Answer from the drawing. Dimensions are ordinates in mm from the lowest x, y and z of the part. Coordinates: 2 decimals unless noted, no trailing zeros. Write each loop counter-clockwise with the first axis right and the second up, starting at its lowest first coordinate (ties: lowest second). Pieces come first, ordered by that corner, then holes.
1) This flat-tipped pin is pushed along its axis until it touches: pin 1 Ø2 at (x, z) = (7.5, 21.5) entering from -Y. Where does it stop, or does it pass through?
2) The part is cut by section C-C (y = 1.25). Determine the outline of the cut face in (x, z), then the cut area to 3 significant figures.
3) The part is cut by section B-B (x = 7.62). Determine the outline of the cut face in (y, z).
4) Find the intervals of material crossed by line 1 (X direction, y = 3.5, z = 12.7); line 2 (Z direction, x = 7.62, y = 2.5); line 3 (X direction, y = 5, z = 9.75), in increasing order.
5) The part is cut by section A-A (z = 12.7). Determine the outline of the cut face in (x, y), then the cut area to 3 significant figures.
6) Determine the mould class of the marked faces 1, 2 and 3 for opening direction X: +X half, -X half, draft (parallel to the pull), parting line (faces both ways), or undercut.
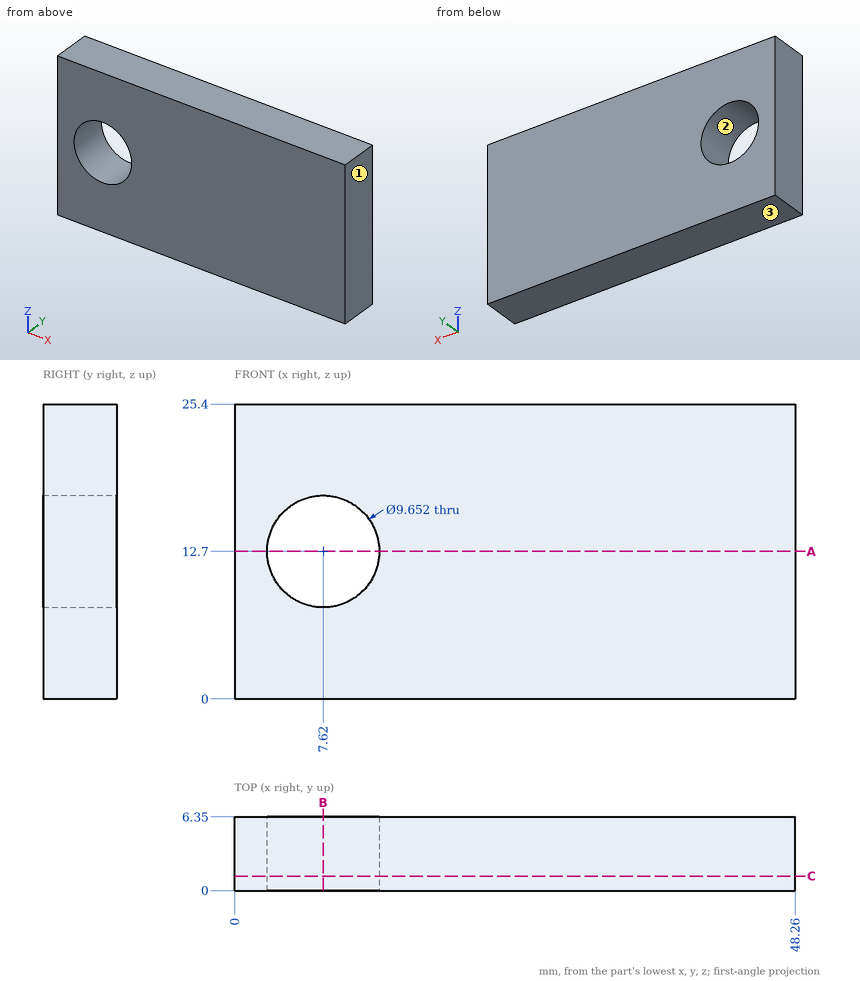
Reported:
1. pin 1: stops at y = 0
2. outline: (0, 0) - (48.26, 0) - (48.26, 25.4) - (0, 25.4) - close; hole circle Ø9.65 at (7.62, 12.7)
2. area: 1,150 mm2
3. outline: (0, 0) - (6.35, 0) - (6.35, 7.87) - (0, 7.87) - close; (0, 17.53) - (6.35, 17.53) - (6.35, 25.4) - (0, 25.4) - close
4. line 1: x = 0 to 2.79, 12.45 to 48.26
4. line 2: z = 0 to 7.87, 17.53 to 25.4
4. line 3: x = 0 to 3.8, 11.44 to 48.26
5. outline: (0, 0) - (2.79, 0) - (2.79, 6.35) - (0, 6.35) - close; (12.45, 0) - (48.26, 0) - (48.26, 6.35) - (12.45, 6.35) - close
5. area: 245 mm2
6. face 1: +X half
6. face 2: undercut
6. face 3: draft
